Autodesk Inventor part; units mm, degrees
ref_plane "YZ Plane" through (0, 0, 0) normal (1, 0, 0) x (0, 1, 0)
ref_plane "XZ Plane" through (0, 0, 0) normal (0, 1, 0) x (-1, 0, 0)
ref_plane "XY Plane" through (0, 0, 0) normal (0, 0, 1) x (1, 0, 0)
sketch "Sketch1" plane through (0, 0, 0) normal (0, 0, 1) x (1, 0, 0)
  line L0 (-12.5, -10) -> (12.5, -10)
  line L1 (12.5, -10) -> (12.5, 10) construction
  line L2 (12.5, 10) -> (-12.5, 10) construction
  line L3 (-12.5, 10) -> (-12.5, -10)
  line L4 (-12.5, -10) -> (12.5, 10) construction
  line L5 (12.5, -10) -> (-12.5, 10)
  line L6 (-12.5, -2.5) -> (-7.5, -2.5)
  line L7 (-7.5, -2.5) -> (-7.5, 2.5) construction
  line L8 (-7.5, 2.5) -> (-12.5, 2.5)
  line L9 (-12.5, 2.5) -> (-12.5, -2.5)
  line L10 (-12.5, -2.5) -> (-7.5, 2.5) construction
  line L11 (-7.5, -2.5) -> (-12.5, 2.5) construction
  line L12 (-7.5, -2.5) -> (-7.5, -10)
  line L13 (-7.5, 2.5) -> (-7.5, 6)
  line L14 (-2.5, -10) -> (2.5, -10)
  line L15 (2.5, -10) -> (2.5, -5)
  line L16 (2.5, -5) -> (-2.5, -5) construction
  line L17 (-2.5, -5) -> (-2.5, -10)
  line L18 (-2.5, -10) -> (2.5, -5) construction
  line L19 (2.5, -10) -> (-2.5, -5) construction
  line L20 (-2.5, -5) -> (-7.5, -5)
  line L21 (2.5, -5) -> (6.25, -5)
  point P0 (0, 0)
  point P1 (-10, 0)
  point P2 (0, 0)
  point P3 (0, -7.5)
  point P4 (2.5, -10)
  dimension "d0" = 20
  dimension "d1" = 25
  dimension "d2" = 5
  dimension "d3" = 5
  dimension "d4" = 10
  dimension "d5" = 5
  dimension "d6" = 5
  dimension "d7" = 12.5
extrude "Extrusion1" add sketch "Sketch1" along normal blind 5 contours L3 L8 L13 L5 L21 L15 L0 L17 L20 L12 L6
equation "\"d5\" = d3"
equation "\"d6\" = d2"
properties part number "camera-bracket-rib"
Read the model definition and answer for the solid it produces. Units are mm, in the model's axes. A direction names the side the tool comes from. Give positions to 0.01 mm unless a question says otherwise; leave off trailing zeros. Write each loop counter-clockwise with the first axis right and the second up, starting at its lowest first coordinate (ties: lowest second). Pieces come first, ordered by that corner, then holes. Notation, with made-up numbers: M 14,81 L 30,81 A23 ccw 30,106 Z; hole C -23.75,-40 d11. An arc over 180 degrees is marked long. Put each result on its own line as item: value. Start each with the question number.
1. Which of the six approach directions +Z, -Z, +X, -X, +Y, -Y give full straight-line access (tool end or side, diameter ignored) to faces 1 (the flat face through (0, -10, 2)), 2 (the flat face through (-10, 2.5, 2)), 3 (the flat face through (-5, -5, 2)), 4 (the flat face through (2.5, -8, 2))?
2. The part is cut by section B-B, the plane x = -5.5. Give the vertices of the cut face in (y, z).
3. The part is cut by section C-C, the plane y = -3. Give the vertices of the cut face in (x, z), and give its area (4 significant figures).
4. Each of these flat-tipped pins is pushed along its axis until it touches: pin 1 Ø2.5 at (x, z) = (-9, 3.5) entering from +Y; pin 2 Ø1 at (y, z) = (4.5, 3.5) entering from -X; pin 3 Ø1.1 at (x, z) = (3.5, 2) entering from -Y. Where does it stop, or does it pass through?
5. The part is cut by section A-A, the plane z = 2.6. Give the vertices of the cut face in (x, y), and give its area (3 significant figures).
6. Consider line 1 along Y through (x, z) = (-9.5, 0.6); line 2 along X through (y, z) = (0, 3.45). Determine where each line is inside the solid, lowest interval first.
Final values:
1. face 1: +Z, -Z, +X, -X, -Y
1. face 2: +Z, -Z, -X, +Y
1. face 3: +Z, -Z, -X, -Y
1. face 4: +Z, -Z, +X, -Y
2. outline: M -5,0 L 4.4,0 L 4.4,5 L -5,5 Z
3. outline: M -7.5,0 L 3.75,0 L 3.75,5 L -7.5,5 Z
3. area: 56.25 mm²
4. pin 1: stops at y = 2.5
4. pin 2: stops at x = -7.5
4. pin 3: stops at y = -5
5. outline: M -12.5,-2.5 L -7.5,-2.5 L -7.5,-5 L -2.5,-5 L -2.5,-10 L 2.5,-10 L 2.5,-5 L 6.25,-5 L -7.5,6 L -7.5,2.5 L -12.5,2.5 Z
5. area: 126 mm²
6. line 1: y = -2.5 to 2.5
6. line 2: x = -12.5 to 0
